Geometry: final body of the model. Coordinates: model frame, mm. A direction names the side the tool comes from. Give positions to 0.01 mm unless a question says otherwise; leave off trailing zeros. Write each loop counter-clockwise with the first axis right and the second up, starting at its lowest first coordinate (ties: lowest second). Pieces come first, ordered by that corner, then holes. Notation, with made-up numbers: (27.5, 77) - (72.5, 77) arc R27 ccw to (72.5, 102) - close; hole circle Ø9 at (28.5, 39.25). An arc over 180 degrees is marked (long way). Return JSON: item names as keys, results as strings.
from build123d import *

# Parameters (mm, degrees)
SKETCH_1_R               = 2.3
EXTRUDE_1_DEPTH          = 1.2
SKETCH_2_R               = 1.5
EXTRUDE_2_DEPTH          = 1.5
CUT_EXTRUDE_1_DEPTH      = 0.5
PATTERN_CIRCULAR_1_COUNT = 20
SKETCH_4_W               = 0.35
SKETCH_4_H               = 0.5
SKETCH_6_W               = 5.3
SKETCH_6_H               = 1.5
CHAMFER_2_SIZE           = 0.5
CUT_EXTRUDE_START        = -0.5
SKETCH_7_R               = 2.3
SKETCH_7_R_2             = 2.1
CUT_EXTRUDE_2_DEPTH      = 0.5


with BuildPart() as part:
    # Эскиз1 → Вытянуть1 (new body)
    with BuildSketch(Plane.XY):
        Circle(SKETCH_1_R)
    extrude(amount=EXTRUDE_1_DEPTH)

    # Эскиз2 → Вытянуть2 (add)
    with BuildSketch(Plane.XY.offset(1.2)):
        Circle(SKETCH_2_R)
    extrude(amount=EXTRUDE_2_DEPTH)

    # Эскиз3 → Вырез-Вытянуть1 (cut)
    with BuildSketch(Plane.XY.offset(1.2)):
        Polygon((-0.33137085, 2.3), (0.33137085, 2.3), (0, 1.5), align=None)
    cut_extrude_1 = extrude(amount=-CUT_EXTRUDE_1_DEPTH, mode=Mode.SUBTRACT)

    # Круговой массив1: Вырез-Вытянуть1 ×20 about axis
    pattern_circular_1_axis = Axis((0, 0, 0), (0, 0, 1))
    for i in range(1, PATTERN_CIRCULAR_1_COUNT):
        add(cut_extrude_1.rotate(pattern_circular_1_axis, i * 360 / PATTERN_CIRCULAR_1_COUNT), mode=Mode.SUBTRACT)

    # Эскиз4 → Вырез-Повернуть1 (revolve, cut)
    with BuildSketch(Plane(origin=(0, 0, 0), x_dir=(1, 0, 0), z_dir=(0, 1, 0))):
        with Locations((1.325, -1.85)):
            Rectangle(SKETCH_4_W, SKETCH_4_H)
    revolve(axis=Axis((0, 0, 10.642619983), (0, 0, -1)), mode=Mode.SUBTRACT)

    # Эскиз6 → Повернуть1 (revolve)
    with BuildSketch(Plane(origin=(0, 0, 0), x_dir=(0, 0, -1), z_dir=(1, 0, 0)), mode=Mode.PRIVATE) as revolve_1_sk:
        with Locations((-5.35, -0.75)):
            Rectangle(SKETCH_6_W, SKETCH_6_H)
    revolve(revolve_1_sk.sketch.rotate(Axis((0, 0, 2.7), (0, 0, 1)), 278.047567557), axis=Axis((0, 0, 2.7), (0, 0, 1)))

    # Фаска2
    # the kernel refuses this chamfer: 0.5 mm, written as the material it takes off along each edge
    with BuildSketch(Plane(origin=(0, 0, 8), x_dir=(-0.9901521845161062, -0.1399951838385265, 0), z_dir=(-0.1399951838385265, 0.9901521845161062, 0))) as chamfer_2_piece_1:
        Polygon((1.5, -CHAMFER_2_SIZE), (1.5 - CHAMFER_2_SIZE, 0), (1.5, 0), align=None)
    revolve(axis=Axis((0, 0, 8), (0, 0, 1)), mode=Mode.SUBTRACT)

    # Эскиз7 → Вырез-Вытянуть2 (cut)
    with BuildSketch(Plane.XY.offset(1.2).offset(CUT_EXTRUDE_START)):
        with Locations(Location((0, 0, 0), (0, 0, 180))):
            Circle(SKETCH_7_R)
        Circle(SKETCH_7_R_2, mode=Mode.SUBTRACT)
    extrude(amount=CUT_EXTRUDE_2_DEPTH, mode=Mode.SUBTRACT)

    # Фаска3
    # the kernel refuses this chamfer: 0.25 mm, written as the material it takes off along each edge
    with BuildSketch(Plane(origin=(0, 0, 2.1), x_dir=(1, 0, 0), z_dir=(0, 1, 0))) as chamfer_3_piece_1:
        with BuildLine():
            Line((1.242928932, 0.007071068), (1.507071068, -0.257071068))
            Line((1.507071068, -0.257071068), (1.512071068, -0.257071068))
            ThreePointArc((1.512071068, -0.257071068), (1.505, -0.128535534), (1.505, 0))
            Line((1.505, 0), (1.5, 0.005))
            ThreePointArc((1.5, 0.005), (1.371464466, 0.005), (1.242928932, 0.012071068))
            Line((1.242928932, 0.012071068), (1.242928932, 0.007071068))
        make_face()
    revolve(axis=Axis((0, 0, 2.1), (0, 0, -1)), mode=Mode.SUBTRACT)


solid = part.part
Q1. Material intervals for probe 1 along Z at (x, y) = (1.65, -0.6); probe 2 along Z at (x, y) = (1.25, -1.1); probe 3 along X at (y, z) = (0.8, 5), sorted ascending. Write a range as [from, to].
Answer key:
{"probe 1": "z = [0, 0.7]", "probe 2": "z = [0, 1.2]", "probe 3": "x = [-1.27, 1.27]"}
Q2. Pin query (flat end, axial travel): P1, Ø0.5, axis at x = -1.5, y = -1, coming from the +Z side; P2, Ø0.6, axis at x = 0.5, y = -1.5, coming from the +Z side; P3, Ø2, axis at y = 1, z = 5.5, coming from the +X side. Return the tip coordinate at first contact, or that it passes through.
Answer key:
{"P1": "stops at z = 1.2", "P2": "stops at z = 7.72", "P3": "stops at x = 1.5"}
Q3. Mould query, pull axis Y, two halves, no side actions, for faces 1 (the cylindrical face through (0.078, -1.498, 4.889)), 2 (the flat face through (0, 0, 8)), 3 (the flat face through (-2, 0, 0.7)). Classes: pulls with the +Y half, pulls with the -Y half, needs draft (parallel to the pull), parting line crosses it, or undercut.
Answer key:
{"face 1": "parting line crosses it", "face 2": "needs draft", "face 3": "undercut"}
Q4. Section query A-A, the plane y = -1.65. Return the cut outline in (x, z), plus the area to 3 significant figures.
Answer key:
{"outline": "(-1.6, 0) - (1.6, 0) - (1.6, 0.7) - (0.99, 0.7) - (0.99, 1.2) - (0.65, 1.2) - (0.65, 0.7) - (0.45, 0.7) - (0.45, 1.2) - (0.06, 1.2) - (0.06, 0.7) - (-0.06, 0.7) - (-0.06, 1.2) - (-0.45, 1.2) - (-0.45, 0.7) - (-0.65, 0.7) - (-0.65, 1.2) - (-0.99, 1.2) - (-0.99, 0.7) - (-1.6, 0.7) - close", "area": "2.96 mm^2"}
Q5. Set-up query: faces 4 (the flat face through (0, 0, 0)), 5 (the cylindrical face through (-0.91, 0.7, 1.85)), 6 (the cylindrical face through (-1.5, 0.07, 1.4)). Return all of +Z, -Z, +X, -X, +Y, -Y with unobstructed straight access to the full face (end or side cutting, diameter ignored); none if empty.
Answer key:
{"face 4": "-Z, +X, -X, +Y, -Y", "face 5": "none", "face 6": "+Z"}
Q6. Section query B-B, the plane z = 3.5. Return the cut outline in (x, y).
Answer key:
{"outline": "circle Ø3 at (0, 0)"}
